Build history of the part. All positions in model axes, mm. Give positions to 0.01 mm unless a question says otherwise; leave off trailing zeros. Loops run counter-clockwise (first coordinate to the right, second up) from the corner with the lowest first, then second, coordinate; pieces in that order, holes last. Notation, with made-up numbers: (-13.5, 89.25) -> (33.5, 89.25) arc R8 cw to (33.5, 99.25) -> close; hole circle Ø9 at (31, 42.25). An arc over 180 degrees is marked (long way). Answer as a JSON object with one key per item and string values. Group by question number.
Q1. Band-saw the part on C-C, the plane x = 7. Write the cut outline in (y, z), plus the area to 3 significant figures.
Q2. Band-saw the part on A-A, the plane y = 3.5. Write the cut outline in (x, z), plus the area to 3 significant figures.
Q3. Wall check: probe 1 along X at (y, z) = (3.25, 0.4); probe 2 along Y at (x, z) = (3, 0.5); probe 3 along X at (y, z) = (-0.25, 0.65). Give the ranges that are in metal, low to high. Write a range as from..to.
Q4. Band-saw the part on B-B, the plane z = 0.35. Write the cut outline in (x, y), plus the area to 3 significant figures.
Q5. Band-saw the part on D-D, the plane y = 0. Write the cut outline in (x, z).
Q6. Drop flat-ended pins along their axis: pin 1 (0.5 mm diameter, centred on y = -0.5, z = 0.5, fed in from -X); pin 2 (3 mm diameter, centred on x = 3.5, y = 1, fed in from +Z). Give the stop position or say it passes through.
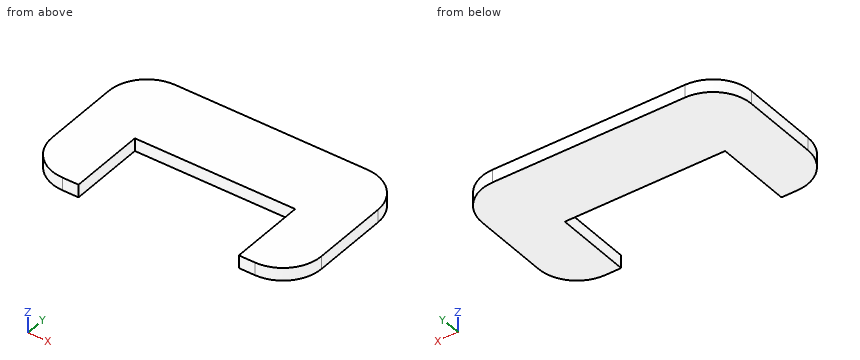
from build123d import *

# Parameters (mm, degrees)
BOSS_EXTRUDE1_DEPTH = 1
FILLET2_R           = 3


with BuildPart() as part:
    # Sketch1 → Boss-Extrude1 (new body)
    with BuildSketch(Plane.XY):
        Polygon((19, 10), (8.5, 10), (8.5, 8), (17, 8), (17, 0), (14.75, 0), (14.75, -2), (19, -2), align=None)
        Polygon((-2, 10), (-2, -2), (2.25, -2), (2.25, 0), (0, 0), (0, 8), (8.5, 8), (8.5, 10), align=None)
        Polygon((0, 0), (2.25, 0), (2.25, 1), (1, 1), (1, 7), (8.5, 7), (8.5, 8), (0, 8), align=None)
        Polygon((1, 1), (2.25, 1), (2.25, 4), (8.5, 4), (8.5, 7), (1, 7), align=None)
        Polygon((16, 7), (8.5, 7), (8.5, 4), (14.75, 4), (14.75, 1), (16, 1), align=None)
        Polygon((17, 8), (8.5, 8), (8.5, 7), (16, 7), (16, 1), (14.75, 1), (14.75, 0), (17, 0), align=None)
    extrude(amount=BOSS_EXTRUDE1_DEPTH)

    # Fillet2
    fillet2_edges = [part.edges().sort_by_distance(p)[0] for p in [
        (-2, -2, 0.5),
        (-2, 10, 0.5),
        (19, 10, 0.5),
        (19, -2, 0.5),
    ]]
    fillet(fillet2_edges, radius=FILLET2_R)


solid = part.part
Worked answers:
{
 "1": {"outline": "(4, 0) -> (10, 0) -> (10, 1) -> (4, 1) -> close", "area": "6.00 mm2"},
 "2": {"outline": "(-2, 0) -> (2.25, 0) -> (2.25, 1) -> (-2, 1) -> close; (14.75, 0) -> (19, 0) -> (19, 1) -> (14.75, 1) -> close", "area": "8.50 mm2"},
 "3": {"probe 1": "-2..2.25, 14.75..19", "probe 2": "4..10", "probe 3": "-1.73..2.25, 14.75..18.73"},
 "4": {"outline": "(-2, 1) arc R3 ccw to (1, -2) -> (2.25, -2) -> (2.25, 4) -> (14.75, 4) -> (14.75, -2) -> (16, -2) arc R3 ccw to (19, 1) -> (19, 7) arc R3 ccw to (16, 10) -> (1, 10) arc R3 ccw to (-2, 7) -> close", "area": "169 mm2"},
 "5": {"outline": "(-1.83, 0) -> (2.25, 0) -> (2.25, 1) -> (-1.83, 1) -> close; (14.75, 0) -> (18.83, 0) -> (18.83, 1) -> (14.75, 1) -> close"},
 "6": {"pin 1": "x = -1.73", "pin 2": "z = 1"}
}
